Input: part model. Units: mm. Frame: model coordinates. A direction names the side the tool comes from. Coordinates: 2 decimals unless noted, no trailing zeros. Order: outer loops, then holes, each group sorted by start corner. A loop starts at its lowest first (then second) coordinate and runs counter-clockwise, first axis right, second up.
from build123d import *

# Parameters (mm, degrees)
PAD002_DEPTH = 57


with BuildPart() as part:
    # Sketch005 → Pad002 (new body)
    with BuildSketch(Plane.YZ):
        with BuildLine():
            Line((-10, 10), (-15, 10))
            Line((-15, 10), (-15, 64.8))
            ThreePointArc((-14.8, 65), (-14.941421, 64.941421), (-15, 64.8))
            Line((-14.8, 65), (-14.5, 65))
            ThreePointArc((-14.374278, 64.814305), (-14.387874, 64.940506), (-14.5, 65))
            Line((-14.411417, 64.721457), (-14.374278, 64.814305))
            ThreePointArc((-14.411417, 64.721457), (-14.477653, 64.495696), (-14.5, 64.261484))
            Line((-14.5, 64.261484), (-14.5, 10.75))
            ThreePointArc((-14.5, 10.75), (-14.426777, 10.573223), (-14.25, 10.5))
            Line((-14.25, 10.5), (-10.75, 10.5))
            ThreePointArc((-10.75, 10.5), (-10.573223, 10.573223), (-10.5, 10.75))
            Line((-10.5, 10.75), (-10.5, 94.75))
            ThreePointArc((-10.5, 94.75), (-10.543246, 94.983405), (-10.667241, 95.185824))
            Line((-14.848271, 99.831412), (-10.667241, 95.185824))
            ThreePointArc((-15, 100.226812), (-14.960766, 100.015056), (-14.848271, 99.831412))
            Line((-15, 102), (-15, 100.226812))
            Line((-15, 102), (-14.5, 102))
            Line((-14.5, 102), (-14.5, 100))
            Line((-14.5, 100), (-10, 95))
            Line((-10, 10), (-10, 95))
        make_face()
    extrude(amount=PAD002_DEPTH)


solid = part.part
Item 1: Cut plane B-B on x = 46. Return loops of the section in (y, z), then the cut area to 3 significant figures.
Response values:
outline: (-15, 10) - (-10, 10) - (-10, 95) - (-14.5, 100) - (-14.5, 102) - (-15, 102) - (-15, 100.23) arc R0.59 ccw to (-14.85, 99.83) - (-10.67, 95.19) arc R0.65 cw to (-10.5, 94.75) - (-10.5, 10.75) arc R0.25 cw to (-10.75, 10.5) - (-14.25, 10.5) arc R0.25 cw to (-14.5, 10.75) - (-14.5, 64.26) arc R1.24 cw to (-14.41, 64.72) - (-14.37, 64.81) arc R0.14 ccw to (-14.5, 65) - (-14.8, 65) arc R0.2 ccw to (-15, 64.8) - close
area: 75.6 mm2
Item 2: Cut plane A-A on z = 35. Return loops of the section in (x, y), then the cut area to 3 significant figures.
Response values:
outline: (0, -15) - (57, -15) - (57, -14.5) - (0, -14.5) - close; (0, -10.5) - (57, -10.5) - (57, -10) - (0, -10) - close
area: 57.0 mm2
Item 3: Cut plane C-C on y = -11.7. Return loops of the section in (x, z), then the cut area to 3 significant figures.
Response values:
outline: (0, 10) - (57, 10) - (57, 10.5) - (0, 10.5) - close; (0, 96.33) - (57, 96.33) - (57, 96.89) - (0, 96.89) - close
area: 60.2 mm2
Item 4: Draft query along Y for faces 1 (the face through (28, -13, 10.5)), 2 (the face through (28.101, -12.282, 97.535)), 3 (the face through (28, -15, 101)). Return one class per face: pulls with the +Y half, pulls with the -Y half, needs draft (parallel to the pull), parting line crosses it, or undercut.
Response values:
face 1: undercut
face 2: pulls with the +Y half
face 3: pulls with the -Y half
Item 5: Access query for faces 4 (the face through (28, -14.5, 101)), 5 (the face through (28, -10.5, 52)), 6 (the face through (57, -14.7, 49.4)), 7 (the face through (28.101, -12.787, 97.541)). Directions: +Z, -Z, +X, -X, +Y, -Y. A direction counts if a zero-diameter tool reaches every point of the face in a straight line with its end or side. Return the directions, or none.
Response values:
face 4: +Z, +X, -X, +Y
face 5: +X, -X
face 6: +Z, -Z, +X, +Y, -Y
face 7: +X, -X, -Y
Item 6: Ray query, probe 1 along Y at (x, z) = (33.5, 62); probe 2 along Z at (x, y) = (48.5, -12.15); probe 3 along Z at (x, y) = (50, -12.05). Return the intervals inside material, ascending.
Response values:
probe 1: y = -15 to -14.5, -10.5 to -10
probe 2: z = 10 to 10.5, 96.83 to 97.39
probe 3: z = 10 to 10.5, 96.72 to 97.28
Item 7: Cut plane D-D on z = 79. Return loops of the section in (x, y).
Response values:
outline: (0, -10.5) - (57, -10.5) - (57, -10) - (0, -10) - close
Item 8: Pin query (flat end, axial travel): pin 1 Ø2 at (x, z) = (21, 101.5) entering from +Y; pin 2 Ø2 at (x, y) = (29, -14) entering from +Z; pin 3 Ø1 at (x, y) = (14.5, -13) entering from +Z; pin 4 Ø3 at (x, y) = (14.5, -11.5) entering from +Z. Return the tip coordinate at first contact, or that it passes through.
Response values:
pin 1: stops at y = -14.5
pin 2: stops at z = 102
pin 3: stops at z = 98.89
pin 4: stops at z = 98.33
